```python
from build123d import *

# Parameters (mm, degrees)
BOSS_EXTRUDE1_DEPTH    = 3.175
CUT_EXTRUDE1_DEPTH     = 233.372048712
FILLET1_R              = 1.27
LPATTERN1_COUNT        = 3
LPATTERN1_PITCH        = 37.3
FILLET1_OF_LPATTERN1_R = 1.27
MIRROR1_START          = -9.743731804
MIRROR1_DEPTH          = 3.175


# Read off the part's stored shape, not the designer's step: Mirror1
with BuildPart() as part:
    # Sketch1 → Boss-Extrude1 (new body)
    with BuildSketch(Plane(origin=(0, -9.743731804, 0), x_dir=(1, 0, 0), z_dir=(0, 1, 0))):
        Polygon((-31.75, 143.175862399), (-28.575, 143.175862399), (-28.575, 171.750862399), (-31.75, 171.750862399), (-31.75, 230.170862399), (31.75, 230.170862399), (31.75, 171.750862399), (28.575, 171.750862399), (28.575, 143.175862399), (31.75, 143.175862399), (31.75, 114.600862399), (28.575, 114.600862399), (28.575, 86.025862399), (31.75, 86.025862399), (31.75, 71.738362399), (-31.75, 71.738362399), (-31.75, 86.025862399), (-28.575, 86.025862399), (-28.575, 114.600862399), (-31.75, 114.600862399), align=None)
        with BuildLine():
            Line((-10.16, 113.330862399), (10.16, 113.330862399))
            ThreePointArc((10.16, 113.330862399), (11.956051224, 112.586913623), (12.7, 110.790862399))
            Line((12.7, 110.790862399), (12.7, 83.870862391))
            ThreePointArc((12.7, 83.870862391), (11.956051224, 82.074811167), (10.16, 81.330862391))
            Line((10.16, 81.330862391), (3.81, 81.330862391))
            Line((3.81, 81.330862391), (3.81, 77.520862391))
            Line((3.81, 77.520862391), (-3.81, 77.520862391))
            Line((-3.81, 77.520862391), (-3.81, 81.330862391))
            Line((-3.81, 81.330862391), (-10.16, 81.330862391))
            ThreePointArc((-10.16, 81.330862391), (-11.956051224, 82.074811167), (-12.7, 83.870862391))
            Line((-12.7, 83.870862391), (-12.7, 110.790862399))
            ThreePointArc((-12.7, 110.790862399), (-11.956051224, 112.586913623), (-10.16, 113.330862399))
        make_face(mode=Mode.SUBTRACT)
    extrude(amount=BOSS_EXTRUDE1_DEPTH)

    # Sketch2 → Cut-Extrude1 (cut, through all)
    with BuildSketch(Plane(origin=(0, -6.568731804, 0), x_dir=(1, 0, 0), z_dir=(0, 1, 0))):
        Polygon((-23.495, 143.810862399), (-23.495, 118.410862399), (-2.54, 118.410862399), align=None)
        Polygon((-23.495, 151.793477209), (-2.54, 126.393477209), (-2.54, 151.793477209), align=None)
    cut_extrude1 = extrude(amount=-CUT_EXTRUDE1_DEPTH, mode=Mode.SUBTRACT)

    # Fillet1
    fillet1_edges = [part.edges().sort_by_distance(p)[0] for p in [
        (-23.495, -8.156231804, -151.793477209),
        (-2.54, -8.156231804, -151.793477209),
        (-2.54, -8.156231804, -126.393477209),
        (-23.495, -8.156231804, -143.810862399),
        (-2.54, -8.156231804, -118.410862399),
        (-23.495, -8.156231804, -118.410862399),
    ]]
    fillet(fillet1_edges, radius=FILLET1_R)

    # LPattern1: Cut-Extrude1 ×3
    with Locations(*[(0, 0, -i * LPATTERN1_PITCH) for i in range(1, LPATTERN1_COUNT)]):
        add(cut_extrude1, mode=Mode.SUBTRACT)

    # Fillet1 of LPattern1
    fillet1_of_lpattern1_edges = [part.edges().sort_by_distance(p)[0] for p in [
        (-23.495, -8.156231804, -189.093477209),
        (-2.54, -8.156231804, -189.093477209),
        (-2.54, -8.156231804, -163.693477209),
        (-23.495, -8.156231804, -181.110862399),
        (-2.54, -8.156231804, -155.710862399),
        (-23.495, -8.156231804, -155.710862399),
        (-23.495, -8.156231804, -226.393477209),
        (-2.54, -8.156231804, -226.393477209),
        (-2.54, -8.156231804, -200.993477209),
        (-23.495, -8.156231804, -218.410862399),
        (-2.54, -8.156231804, -193.010862399),
        (-23.495, -8.156231804, -193.010862399),
    ]]
    fillet(fillet1_of_lpattern1_edges, radius=FILLET1_OF_LPATTERN1_R)

    # Mirror1 outline → Mirror1 (cut)
    with BuildSketch(Plane(origin=(0, 0, 0), x_dir=(1, 0, 0), z_dir=(0, 1, 0)).offset(MIRROR1_START)):
        with BuildLine():
            Line((20.800835695, 226.393477209), (3.81, 226.393477209))
            ThreePointArc((3.81, 226.393477209), (2.911974388, 226.021502821), (2.54, 225.123477209))
            Line((2.54, 225.123477209), (2.54, 204.528524851))
            ThreePointArc((2.54, 204.528524851), (3.380609712, 203.333316091), (4.789644064, 203.720318499))
            Line((4.789644064, 203.720318499), (21.780479759, 224.315270857))
            ThreePointArc((21.780479759, 224.315270857), (21.949600699, 225.664992644), (20.800835695, 226.393477209))
        make_face()
        with BuildLine():
            Line((5.234164305, 193.010862399), (22.225, 193.010862399))
            ThreePointArc((22.225, 193.010862399), (23.123025612, 193.382836787), (23.495, 194.280862399))
            Line((23.495, 194.280862399), (23.495, 214.875814757))
            ThreePointArc((23.495, 214.875814757), (22.654390288, 216.071023517), (21.245355936, 215.68402111))
            Line((21.245355936, 215.68402111), (4.254520241, 195.089068752))
            ThreePointArc((4.254520241, 195.089068752), (4.085399301, 193.739346964), (5.234164305, 193.010862399))
        make_face()
        with BuildLine():
            Line((5.234164305, 118.410862399), (22.225, 118.410862399))
            ThreePointArc((22.225, 118.410862399), (23.123025612, 118.782836787), (23.495, 119.680862399))
            Line((23.495, 119.680862399), (23.495, 140.275814757))
            ThreePointArc((23.495, 140.275814757), (22.654390288, 141.471023517), (21.245355936, 141.08402111))
            Line((21.245355936, 141.08402111), (4.254520241, 120.489068752))
            ThreePointArc((4.254520241, 120.489068752), (4.085399301, 119.139346964), (5.234164305, 118.410862399))
        make_face()
        with BuildLine():
            Line((20.800835695, 151.793477209), (3.81, 151.793477209))
            ThreePointArc((3.81, 151.793477209), (2.911974388, 151.421502821), (2.54, 150.523477209))
            Line((2.54, 150.523477209), (2.54, 129.928524851))
            ThreePointArc((2.54, 129.928524851), (3.380609712, 128.733316091), (4.789644064, 129.120318499))
            Line((4.789644064, 129.120318499), (21.780479759, 149.715270857))
            ThreePointArc((21.780479759, 149.715270857), (21.949600699, 151.064992644), (20.800835695, 151.793477209))
        make_face()
        with BuildLine():
            Line((5.234164305, 155.710862399), (22.225, 155.710862399))
            ThreePointArc((22.225, 155.710862399), (23.123025612, 156.082836787), (23.495, 156.980862399))
            Line((23.495, 156.980862399), (23.495, 177.575814757))
            ThreePointArc((23.495, 177.575814757), (22.654390288, 178.771023517), (21.245355936, 178.38402111))
            Line((21.245355936, 178.38402111), (4.254520241, 157.789068752))
            ThreePointArc((4.254520241, 157.789068752), (4.085399301, 156.439346964), (5.234164305, 155.710862399))
        make_face()
        with BuildLine():
            Line((20.800835695, 189.093477209), (3.81, 189.093477209))
            ThreePointArc((3.81, 189.093477209), (2.911974388, 188.721502821), (2.54, 187.823477209))
            Line((2.54, 187.823477209), (2.54, 167.228524851))
            ThreePointArc((2.54, 167.228524851), (3.380609712, 166.033316091), (4.789644064, 166.420318499))
            Line((4.789644064, 166.420318499), (21.780479759, 187.015270857))
            ThreePointArc((21.780479759, 187.015270857), (21.949600699, 188.364992644), (20.800835695, 189.093477209))
        make_face()
    extrude(amount=MIRROR1_DEPTH, mode=Mode.SUBTRACT)


solid = part.part
```
Check sheet for the modelled part. Datum: model origin and axes. Units: mm. A direction names the side the tool comes from. Give positions to 0.01 mm unless a question says otherwise; leave off trailing zeros. Write each loop counter-clockwise with the first axis right and the second up, starting at its lowest first coordinate (ties: lowest second). Pieces come first, ordered by that corner, then holes.
Item 1: Cross-section at B-B (z = -92). Enter the section's corners in (x, y) (3 decimals).
Item 2: Scan lines: L1, parallel to X at y = -9.35, z = -206.5 (3 decimals); L2, parallel to X at y = -8.4, z = -199 (3 decimals); L3, parallel to X at y = -7.25, z = -175.5 (3 decimals). Record each from-to range of solid material in increasing order.
Item 3: Cross-section at D-D (z = -183). Enter the section's corners in (x, y), and give its area (3 significant figures).
Item 4: Cross-section at C-C (x = -18.5). Enter the section's corners in (y, z), and give its area (3 significant figures).
Item 5: Access from +Z, -Z, +X, -X, +Y, -Y to the whole of each face (thin tool, end or side, straight path). Record for faces 1 (the face through (-23.495, -8, -167)), 2 (the face through (28.575, -8, -158)), 3 (the face through (-30, -8, -143.176)).
Item 6: Cross-section at A-A (x = -0.5). Enter the section's corners in (y, z), and give its area (3 significant figures).
Report:
1. outline: (-28.575, -9.744) - (-12.7, -9.744) - (-12.7, -6.569) - (-28.575, -6.569) - close; (12.7, -9.744) - (28.575, -9.744) - (28.575, -6.569) - (12.7, -6.569) - close
2. L1: x = -31.75 to -23.495, -13.669 to -7.083, -2.54 to 2.54, 7.083 to 13.669, 23.495 to 31.75
2. L2: x = -31.75 to -23.495, -7.481 to 7.481, 23.495 to 31.75
2. L3: x = -31.75 to -23.495, -18.866 to -12.28, -2.54 to 2.54, 12.28 to 18.866, 23.495 to 31.75
3. outline: (-31.75, -9.74) - (-18.47, -9.74) - (-18.47, -6.57) - (-31.75, -6.57) - close; (-2.54, -9.74) - (2.54, -9.74) - (2.54, -6.57) - (-2.54, -6.57) - close; (18.47, -9.74) - (31.75, -9.74) - (31.75, -6.57) - (18.47, -6.57) - close
3. area: 100 mm2
4. outline: (-9.74, -230.17) - (-6.57, -230.17) - (-6.57, -226.39) - (-9.74, -226.39) - close; (-9.74, -220.34) - (-6.57, -220.34) - (-6.57, -212.36) - (-9.74, -212.36) - close; (-9.74, -193.01) - (-6.57, -193.01) - (-6.57, -189.09) - (-9.74, -189.09) - close; (-9.74, -183.04) - (-6.57, -183.04) - (-6.57, -175.06) - (-9.74, -175.06) - close; (-9.74, -155.71) - (-6.57, -155.71) - (-6.57, -151.79) - (-9.74, -151.79) - close; (-9.74, -145.74) - (-6.57, -145.74) - (-6.57, -137.76) - (-9.74, -137.76) - close; (-9.74, -118.41) - (-6.57, -118.41) - (-6.57, -71.74) - (-9.74, -71.74) - close
4. area: 261 mm2
5. face 1: +Y, -Y
5. face 2: +X, +Y, -Y
5. face 3: -X, +Y, -Y
6. outline: (-9.74, -230.17) - (-6.57, -230.17) - (-6.57, -113.33) - (-9.74, -113.33) - close; (-9.74, -77.52) - (-6.57, -77.52) - (-6.57, -71.74) - (-9.74, -71.74) - close
6. area: 389 mm2
